Autodesk Inventor part; units mm, degrees
ref_plane "YZ Plane" through (0, 0, 0) normal (1, 0, 0) x (0, 1, 0)
ref_plane "XZ Plane" through (0, 0, 0) normal (0, 1, 0) x (-1, 0, 0)
ref_plane "XY Plane" through (0, 0, 0) normal (0, 0, 1) x (1, 0, 0)
sketch "Sketch7" plane through (0, 0, 0) normal (0, 1, 0) x (-1, 0, 0)
  line L0 (12.7, 6.35) -> (4.0386, 6.35)
  line L1 (-12.7, 6.35) -> (-12.7, -6.35)
  line L2 (-12.7, -6.35) -> (-4.0386, -6.35)
  line L3 (12.7, -6.35) -> (12.7, 6.35)
  line L4 (12.7, 6.35) -> (-12.7, -6.35) construction
  line L5 (-12.7, 6.35) -> (12.7, -6.35) construction
  line L6 (8.6614, 2.3114) -> (4.0386, 2.3114)
  line L7 (4.0386, 2.3114) -> (4.0386, -2.3114)
  line L8 (4.0386, -2.3114) -> (8.6614, -2.3114)
  line L9 (8.6614, -2.3114) -> (8.6614, 2.3114)
  line L10 (8.6614, 2.3114) -> (4.0386, -2.3114) construction
  line L11 (4.0386, 2.3114) -> (8.6614, -2.3114) construction
  line L12 (-8.6614, 2.3114) -> (-4.0386, 2.3114)
  line L13 (-4.0386, 2.3114) -> (-4.0386, -2.3114)
  line L14 (-4.0386, -2.3114) -> (-8.6614, -2.3114)
  line L15 (-8.6614, -2.3114) -> (-8.6614, 2.3114)
  line L16 (-8.6614, 2.3114) -> (-4.0386, -2.3114) construction
  line L17 (-4.0386, 2.3114) -> (-8.6614, -2.3114) construction
  line L18 (4.0386, 6.35) -> (4.0386, 11.43)
  line L19 (4.0386, 11.43) -> (-4.0386, 11.43)
  line L20 (-4.0386, 11.43) -> (-4.0386, 6.35)
  line L21 (-4.0386, -6.35) -> (-4.0386, -11.43)
  line L22 (-4.0386, -11.43) -> (4.0386, -11.43)
  line L23 (4.0386, -11.43) -> (4.0386, -6.35)
  line L24 (-4.0386, 6.35) -> (-12.7, 6.35)
  line L25 (4.0386, -6.35) -> (12.7, -6.35)
  point P0 (0, 0)
  point P1 (6.35, 0)
  point P2 (-6.35, 0)
  dimension "d29" = 25.4
  dimension "d30" = 12.7
  dimension "d31" = 4.6228
  dimension "d32" = 4.6228
  dimension "d33" = 4.6228
  dimension "d34" = 4.6228
  dimension "d35" = 12.7
  dimension "d36" = 6.35
  dimension "d37" = 5.08
  dimension "d40" = 5.08
extrude "Extrusion2" add sketch "Sketch7" along normal blind 1.1684
sketch "Sketch8" plane through (0, 1.1684, 0) normal (0, 1, 0) x (1, 0, 0)
  circle A0 centre (0, -6.35) radius 2.4003
  point P0 (0, 0)
  dimension "d47" = 4.8006
  dimension "d49" = 6.35
sketch "Sketch9" plane through (0, 1.1684, 0) normal (0, 1, 0) x (1, 0, 0)
  circle A0 centre (0, 6.35) radius 2.4003
  point P0 (0, 0)
  dimension "d51" = 4.8006
  dimension "d52" = 6.35
extrude "Extrusion3" add sketch "Sketch8" along normal blind 8.001
extrude "Extrusion4" add sketch "Sketch9" along normal blind 8.001
properties part number "VexLegoWidget"
The listing builds one solid part. Answer for the finished solid, in the listing's coordinates (mm). A direction names the side the tool comes from. Round coordinates to 2 decimals unless told otherwise and drop trailing zeros. Loops run counter-clockwise (first coordinate to the right, second up) from the corner with the lowest first, then second, coordinate; pieces in that order, holes last. Notation, with made-up numbers: (-20.5, -35.5) -> (-4.5, -35.5) arc R25 cw to (-4.5, -14.5) -> close; hole circle Ø2 at (-12, 32). An arc over 180 degrees is marked (long way). Use one line per item in the form item = value.
1. The part is cut by section C-C on x = 0. Determine the outline of the cut face in (y, z).
Answer key:
outline = (0, -11.43) -> (1.17, -11.43) -> (1.17, -8.75) -> (9.17, -8.75) -> (9.17, -3.95) -> (1.17, -3.95) -> (1.17, 3.95) -> (9.17, 3.95) -> (9.17, 8.75) -> (1.17, 8.75) -> (1.17, 11.43) -> (0, 11.43) -> close
2. The part is cut by section A-A on x = 6. Determine the outline of the cut face in (y, z), and give its area (3 significant figures).
Answer key:
outline = (0, -6.35) -> (1.17, -6.35) -> (1.17, -2.31) -> (0, -2.31) -> close; (0, 2.31) -> (1.17, 2.31) -> (1.17, 6.35) -> (0, 6.35) -> close
area = 9.44 mm²
3. Find the intervals of material crossed by probe 1 along X at (y, z) = (1, -1.5); probe 2 along Y at (x, z) = (-1.75, 0.75); probe 3 along X at (y, z) = (4, 6.5), in increasing order. Write a range as [from, to].
Answer key:
probe_1 = [-12.7, -8.66], [-4.04, 4.04], [8.66, 12.7]
probe_2 = [0, 1.17]
probe_3 = [-2.4, 2.4]
4. A tool of negligible diameter and unlimited length cuts with its end or side. For faces 1 (the flat face through (-4.039, 1, -9)), 2 (the flat face through (6, 1, 2.311)), 3 (the cylindrical face through (-0.52, 5.113, -8.693)), 4 (the flat face through (0, 9.169, -6)), 5 (the flat face through (4.039, 1, -9)), from which of +Z, -Z, +X, -X, +Y, -Y can it reach the whole face along a straight path? Write none if from no direction.
Answer key:
face_1 = -Z, -X, +Y, -Y
face_2 = +Y, -Y
face_3 = +Y
face_4 = +Z, -Z, +X, -X, +Y
face_5 = -Z, +X, +Y, -Y
5. The part is cut by section D-D on z = -8. Determine the outline of the cut face in (x, y), and give its area (3 significant figures).
Answer key:
outline = (-4.04, 0) -> (4.04, 0) -> (4.04, 1.17) -> (1.74, 1.17) -> (1.74, 9.17) -> (-1.74, 9.17) -> (-1.74, 1.17) -> (-4.04, 1.17) -> close
area = 37.3 mm²
6. Flat-ended cylindrical pins translate along their axes: pin 1 Ø1.3 at (x, y) = (-10.5, 0.5) entering from -Z; pin 2 Ø1.3 at (y, z) = (0.5, -9) entering from +X; pin 3 Ø0.6 at (x, y) = (-8, 1) entering from +Z; pin 4 Ø1 at (x, y) = (-4, 7.5) entering from +Z. Find the tip coordinate at first contact, or state that the pin passes through.
Answer key:
pin_1 = -6.35
pin_2 = 4.04
pin_3 = 6.35
pin_4 = through
7. The part is cut by section B-B on y = 8. Determine the outline of the cut face in (x, z), and give its area (3 significant figures).
Answer key:
outline = circle Ø4.8 at (0, -6.35); circle Ø4.8 at (0, 6.35)
area = 36.2 mm²
8. For a pull along X with two mould halves and no side action, classify faces 6 (the flat face through (4.039, 1, 9)), 7 (the cylindrical face through (-0.31, 5.11, 8.73)), 8 (the flat face through (0, 1, 11.43)), 9 (the flat face through (-8.661, 1, 0)) as released by +X, released by -X, zero draft, split by the parting line, or undercut.
Answer key:
face_6 = released by +X
face_7 = split by the parting line
face_8 = zero draft
face_9 = undercut
